Work out the finished part from the listing and answer in its coordinate system (mm). A direction names the side the tool comes from. Coordinates: 2 decimals unless noted, no trailing zeros. Write each loop counter-clockwise with the first axis right and the second up, starting at its lowest first coordinate (ties: lowest second). Pieces come first, ordered by that corner, then holes. Notation, with made-up numbers: (25.5, -7.75) - (73.5, -7.75) arc R21 cw to (73.5, 6.25) - close; hole circle Ø11 at (-28, -17.5). An arc over 180 degrees is marked (long way). Answer as a JSON object with one key per item and string values. Group by question number.
from build123d import *

# Parameters (mm, degrees)
SKICA1_W                 = 30
SKICA1_H                 = 30
SKICA1_R                 = 1.5
P_IDAT_VYSUNUT_M1_DEPTH  = 7
SKICA2_W                 = 30
SKICA2_H                 = 30
P_IDAT_VYSUNUT_M2_DEPTH  = 11
SKICA3_W                 = 7
SKICA3_H                 = 2
ODEBRAT_VYSUNUT_M1_DEPTH = 30
SKICA4_R                 = 1.5
P_IDAT_VYSUNUT_M3_DEPTH  = 3.5
SKICA5_W                 = 16
SKICA5_H                 = 20
P_IDAT_VYSUNUT_M4_DEPTH  = 11.5
P_IDAT_VYSUNUT_M5_DEPTH  = 6.5
ZKOSEN_1_SIZE            = 3


with BuildPart() as part:
    # Skica1 → Přidat vysunutím1 (new body)
    with BuildSketch(Plane.XY):
        Rectangle(SKICA1_W, SKICA1_H)
        with Locations((5, 5)):
            Circle(SKICA1_R, mode=Mode.SUBTRACT)
        with Locations((-5, 5)):
            Circle(SKICA1_R, mode=Mode.SUBTRACT)
        with Locations((0, -5)):
            Circle(SKICA1_R, mode=Mode.SUBTRACT)
    extrude(amount=P_IDAT_VYSUNUT_M1_DEPTH)

    # Skica2 → Přidat vysunutím2 (add)
    with BuildSketch(Plane.XY.offset(7)):
        Rectangle(SKICA2_W, SKICA2_H)
    extrude(amount=P_IDAT_VYSUNUT_M2_DEPTH)

    # Skica3 → Odebrat vysunutím1 (cut)
    with BuildSketch(Plane(origin=(15, 0, 0), x_dir=(0, 0, -1), z_dir=(1, 0, 0))):
        with Locations((-14.5, 12)):
            Rectangle(SKICA3_W, SKICA3_H)
        with Locations((-14.5, 8)):
            Rectangle(SKICA3_W, SKICA3_H)
        with Locations((-14.5, 4)):
            Rectangle(SKICA3_W, SKICA3_H)
        with Locations((-14.5, 0)):
            Rectangle(SKICA3_W, SKICA3_H)
        with Locations((-14.5, -4)):
            Rectangle(SKICA3_W, SKICA3_H)
        with Locations((-14.5, -8)):
            Rectangle(SKICA3_W, SKICA3_H)
        with Locations((-14.5, -12)):
            Rectangle(SKICA3_W, SKICA3_H)
    extrude(amount=-ODEBRAT_VYSUNUT_M1_DEPTH, mode=Mode.SUBTRACT)

    # Skica4 → Přidat vysunutím3 (add)
    with BuildSketch(Plane.XZ.offset(15)):
        with Locations(Location((9, 6, 0), (0, 0, 180))):
            Circle(SKICA4_R)
        with Locations(Location((-9, 6, 0), (0, 0, 180))):
            Circle(SKICA4_R)
    extrude(amount=P_IDAT_VYSUNUT_M3_DEPTH)

    # Skica5 → Přidat vysunutím4 (add)
    with BuildSketch(Plane.XZ.offset(18.5)):
        with Locations((9, 11)):
            Rectangle(SKICA5_W, SKICA5_H)
        with Locations((-9, 11)):
            Rectangle(SKICA5_W, SKICA5_H)
    extrude(amount=P_IDAT_VYSUNUT_M4_DEPTH)

    # Skica6 → Přidat vysunutím5 (add)
    with BuildSketch(Plane.XZ.offset(30)):
        Polygon((-4.958548116, 6), (-6.979274058, 9.5), (-11.020725942, 9.5), (-13.041451884, 6), (-11.020725942, 2.5), (-6.979274058, 2.5), align=None)
        Polygon((6.979274058, 2.5), (4.958548116, 6), (6.979274058, 9.5), (11.020725942, 9.5), (13.041451884, 6), (11.020725942, 2.5), align=None)
    extrude(amount=P_IDAT_VYSUNUT_M5_DEPTH)

    # Zkosení1
    zkosen_1_edges = [part.edges().sort_by_distance(p)[0] for p in [
        (-5.968911087, -36.5, 4.25),
        (-5.968911087, -36.5, 7.75),
        (-9, -36.5, 9.5),
        (-12.031088913, -36.5, 7.75),
        (-12.031088913, -36.5, 4.25),
        (-9, -36.5, 2.5),
        (9, -36.5, 2.5),
        (12.031088913, -36.5, 4.25),
        (12.031088913, -36.5, 7.75),
        (9, -36.5, 9.5),
        (5.968911087, -36.5, 7.75),
        (5.968911087, -36.5, 4.25),
    ]]
    chamfer(zkosen_1_edges, length=ZKOSEN_1_SIZE)


solid = part.part
Q1. Section A-A on z = 3.5 is taken. Determine the outline of the cut face in (x, y).
Q2. Section B-B on z = 14.25 is taken. Count the separate pieces of the cut face and the enclosed holes in it, plus the area to 3 significant figures.
Q3. Consider L1, parallel to Y at x = 5, z = 4.5; L2, parallel to X at y = -23, z = 4; L3, parallel to Z at x = 6, y = 11.5. Determine where each line is inside the solid, lowest interval first. Write a range as from..to.
Q4. A tool of negligible diameter and unlimited length cuts with its end or side. For faces 4 (the face through (0, -6, 18)), 5 (the face through (0, 13, 15)), 6 (the face through (9, -24, 1)), from which of +Z, -Z, +X, -X, +Y, -Y can it reach the whole face along a straight path? Write none if from no direction.
Q5. Flat-ended cylindrical pins translate along their axes: pin 1 Ø5 at (y, z) = (-4.5, 4) entering from -X; pin 2 Ø1.6 at (x, y) = (3.5, 4) entering from +Z; pin 3 Ø1.6 at (x, y) = (-3.5, 5.5) entering from +Z. Find the tip coordinate at first contact, or state that the pin passes through.
Q6. For a pull along X with two mould halves and no side action, classify faces 1 (the face through (7.012, -34.688, 4.819)), 2 (the face through (0, 14, 18)), 3 (the face through (-10.988, -34.688, 7.181)) as +X half, -X half, draft (parallel to the pull), parting line (faces both ways), or undercut.
Numbers:
{
 "1": {"outline": "(-17, -30) - (-11.6, -30) - (-11.6, -33.5) - (-10.44, -34.5) - (-7.56, -34.5) - (-6.4, -33.5) - (-6.4, -30) - (-1, -30) - (-1, -18.5) - (-17, -18.5) - close; (-15, -15) - (15, -15) - (15, 15) - (-15, 15) - close; (1, -30) - (6.4, -30) - (6.4, -33.5) - (7.56, -34.5) - (10.44, -34.5) - (11.6, -33.5) - (11.6, -30) - (17, -30) - (17, -18.5) - (1, -18.5) - close; hole circle Ø3 at (-5, 5); hole circle Ø3 at (0, -5); hole circle Ø3 at (5, 5)"},
 "2": {"separate pieces": "10", "enclosed holes": "0", "area": "848 mm²"},
 "3": {"L1": "y = -30..-18.5, -15..3.5, 6.5..15", "L2": "x = -17..-1, 1..17", "L3": "z = 0..11"},
 "4": {"face 4": "+Z, +X, -X, +Y", "face 5": "+Z, +X, -X", "face 6": "-Z, +X, -X, -Y"},
 "5": {"pin 1": "stops at x = -15", "pin 2": "stops at z = 11", "pin 3": "stops at z = 18"},
 "6": {"face 1": "undercut", "face 2": "draft", "face 3": "-X half"}
}
